```python
from build123d import *

# Parameters (mm, degrees)
SKETCH1_R           = 4.7625
SKETCH1_R_2         = 2.49555
BOSS_EXTRUDE1_DEPTH = 6.35
CUT_EXTRUDE1_START  = -5.08
SKETCH2_R           = 4.7625
SKETCH2_R_2         = 3.96875
CUT_EXTRUDE1_DEPTH  = 3.81


with BuildPart() as part:
    # Sketch1 → Boss-Extrude1 (new body)
    with BuildSketch(Plane(origin=(0, 0, 0), x_dir=(1, 0, 0), z_dir=(0, 1, 0))):
        Circle(SKETCH1_R)
        Circle(SKETCH1_R_2, mode=Mode.SUBTRACT)
    extrude(amount=BOSS_EXTRUDE1_DEPTH)

    # Sketch2 → Cut-Extrude1 (cut)
    with BuildSketch(Plane(origin=(0, 6.35, 0), x_dir=(1, 0, 0), z_dir=(0, 1, 0)).offset(CUT_EXTRUDE1_START)):
        Circle(SKETCH2_R)
        Circle(SKETCH2_R_2, mode=Mode.SUBTRACT)
    extrude(amount=CUT_EXTRUDE1_DEPTH, mode=Mode.SUBTRACT)


solid = part.part
```
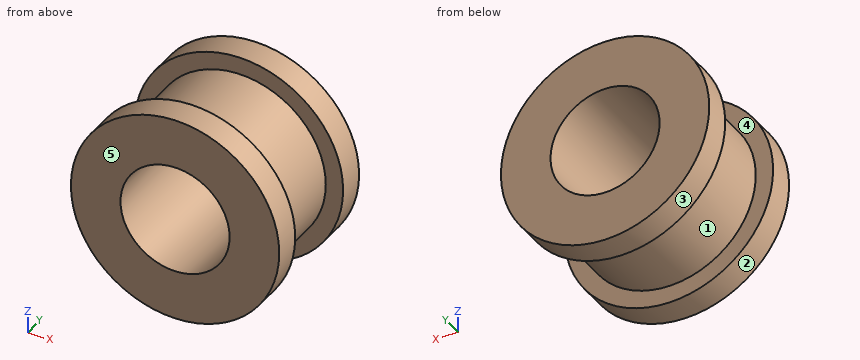
Check sheet for the modelled part. Datum: model origin and axes. Units: mm. Face numbers are marked on the shaded views. A direction names the side the tool comes from. Round coordinates to 2 decimals unless told otherwise and drop trailing zeros. Loops run counter-clockwise (first coordinate to the right, second up) from the corner with the lowest first, then second, coordinate; pieces in that order, holes last. Notation, with made-up numbers: M 28,46.25 L 42,46.25 A25 cw 42,73.25 Z; hole C 40.5,34 d4. An arc over 180 degrees is marked long. Answer as a JSON object with one key per item and string values.
1. Section check C-C (y = 0.5). Record the boundary of the cut face in (x, z) (1 decimal), plus the area to 3 significant figures.
Reply:
{"outline": "C 0,0 d9.5; hole C 0,0 d5", "area": "51.7 mm²"}
2. Access from +Z, -Z, +X, -X, +Y, -Y to the whole of each face (thin tool, end or side, straight path). Record for the marked faces 1 and 2.
Reply:
{"face 1": "none", "face 2": "+Y, -Y"}
3. Section check A-A (x = 0). Record the boundary of the cut face in (y, z), plus the area to 3 significant figures.
Reply:
{"outline": "M 0,-4.76 L 1.27,-4.76 L 1.27,-3.97 L 5.08,-3.97 L 5.08,-4.76 L 6.35,-4.76 L 6.35,-2.5 L 0,-2.5 Z; M 0,2.5 L 6.35,2.5 L 6.35,4.76 L 5.08,4.76 L 5.08,3.97 L 1.27,3.97 L 1.27,4.76 L 0,4.76 Z", "area": "22.7 mm²"}
4. Section check B-B (z = 0). Record the boundary of the cut face in (x, y), plus the area to 3 significant figures.
Reply:
{"outline": "M -4.76,0 L -2.5,0 L -2.5,6.35 L -4.76,6.35 L -4.76,5.08 L -3.97,5.08 L -3.97,1.27 L -4.76,1.27 Z; M 2.5,0 L 4.76,0 L 4.76,1.27 L 3.97,1.27 L 3.97,5.08 L 4.76,5.08 L 4.76,6.35 L 2.5,6.35 Z", "area": "22.7 mm²"}
5. Gauge pin test, flat ends, axial feed: P1, Ø1.5, axis at x = -2, z = 1, coming from the +Y side; P2, Ø3, axis at y = 4.5, z = 1.5, coming from the -X side; P3, Ø1.5, axis at y = 2.5, z = -1, coming from the -X side; P4, Ø2, axis at y = 2.5, z = 3, coming from the -X side. Record the tip position at first contact, or that the pin passes through.
Reply:
{"P1": "stops at y = 6.35", "P2": "stops at x = -4.76", "P3": "stops at x = -3.96", "P4": "stops at x = -3.43"}
6. Mould release check, pull along Y, two halves, no side actions. Record for the marked faces 3, 4 and 5: pulls with the +Y half, pulls with the -Y half, needs draft (parallel to the pull), parting line crosses it, or undercut.
Reply:
{"face 3": "needs draft", "face 4": "undercut", "face 5": "pulls with the -Y half"}
7. Section check D-D (x = -3.5). Record the boundary of the cut face in (y, z), plus the area to 3 significant figures.
Reply:
{"outline": "M 0,-3.23 L 1.27,-3.23 L 1.27,-1.87 L 5.08,-1.87 L 5.08,-3.23 L 6.35,-3.23 L 6.35,3.23 L 5.08,3.23 L 5.08,1.87 L 1.27,1.87 L 1.27,3.23 L 0,3.23 Z", "area": "30.7 mm²"}
8. Scan lines: line 1 (Y direction, x = 4.5, z = 0.5); line 2 (X direction, y = 2.75, z = 0). Record each from-to range of solid material in increasing order.
Reply:
{"line 1": "y = 0 to 1.27, 5.08 to 6.35", "line 2": "x = -3.97 to -2.5, 2.5 to 3.97"}
